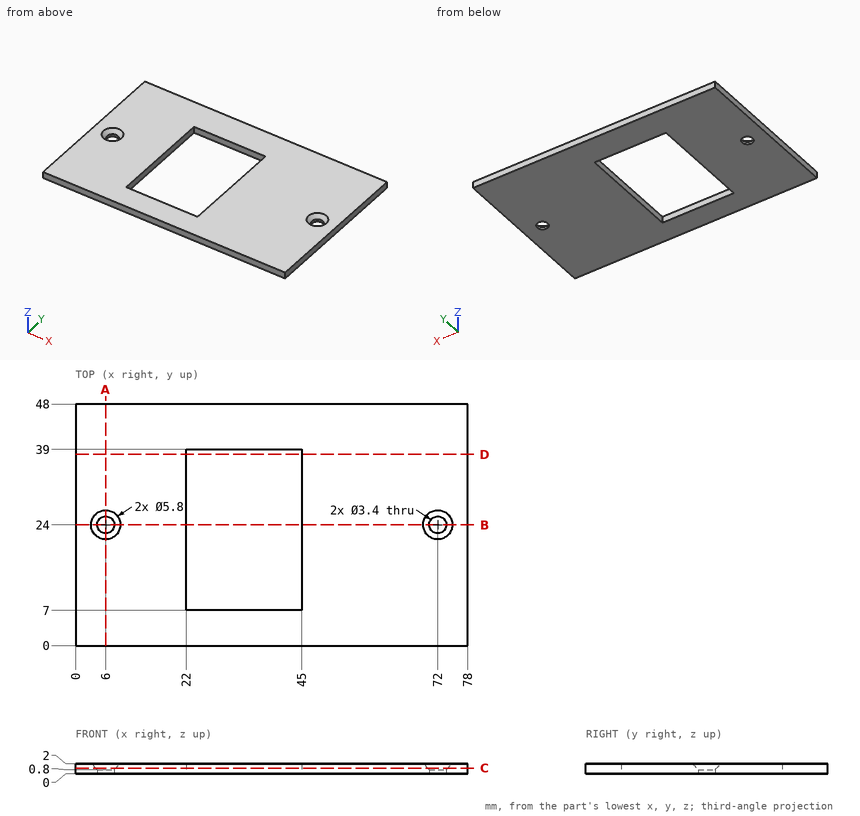
Input: dimensioned drawing with shaded views. Units: mm. Origin: part minimum x, y, z. Give positions to 0.01 mm unless a question says otherwise; leave off trailing zeros. Write each loop counter-clockwise with the first axis right and the second up, starting at its lowest first coordinate (ties: lowest second). Pieces come first, ordered by that corner, then holes. Notation, with made-up numbers: (48.25, 45) -> (68.25, 45) arc R20 cw to (68.25, 68) -> close; hole circle Ø1 at (43, 41). An arc over 180 degrees is marked (long way). Return JSON: item names as keys, results as strings. Group by question number.
1. Section B-B, the plane y = 24. Output: boundary loops of the cut face in (x, z).
2. Section D-D, the plane y = 38. Output: boundary loops of the cut face in (x, z), then the cut area to 3 significant figures.
3. Section C-C, the plane z = 1.1. Output: boundary loops of the cut face in (x, y), then the cut area to 3 significant figures.
4. Pin query (flat end, axial travel): pin 1 Ø10 at (x, y) = (13.5, 23.5) entering from -Z; pin 2 Ø5.5 at (x, y) = (72, 24) entering from +Z. Return the tip coordinate at first contact, or that it passes through.
5. Material intervals for line 1 (X direction, y = 24, z = 0.2); line 2 (Y direction, x = 6, z = 0.55); line 3 (Y direction, x = 37.5, z = 1.4), sorted ascending. Write a range as from..to.
6. Section A-A, the plane x = 6. Output: boundary loops of the cut face in (y, z), then the cut area to 3 significant figures.
Determined:
{
 "1": {"outline": "(0, 0) -> (4.3, 0) -> (4.3, 0.8) -> (3.1, 2) -> (0, 2) -> close; (7.7, 0) -> (22, 0) -> (22, 2) -> (8.9, 2) -> (7.7, 0.8) -> close; (45, 0) -> (70.3, 0) -> (70.3, 0.8) -> (69.1, 2) -> (45, 2) -> close; (73.7, 0) -> (78, 0) -> (78, 2) -> (74.9, 2) -> (73.7, 0.8) -> close"},
 "2": {"outline": "(0, 0) -> (22, 0) -> (22, 2) -> (0, 2) -> close; (45, 0) -> (78, 0) -> (78, 2) -> (45, 2) -> close", "area": "110 mm2"},
 "3": {"outline": "(0, 0) -> (78, 0) -> (78, 48) -> (0, 48) -> close; hole circle Ø4 at (6, 24); hole (22, 7) -> (45, 7) -> (45, 39) -> (22, 39) -> close; hole circle Ø4 at (72, 24)", "area": "2,980 mm2"},
 "4": {"pin 1": "stops at z = 0", "pin 2": "stops at z = 1.85"},
 "5": {"line 1": "x = 0..4.3, 7.7..22, 45..70.3, 73.7..78", "line 2": "y = 0..22.3, 25.7..48", "line 3": "y = 0..7, 39..48"},
 "6": {"outline": "(0, 0) -> (22.3, 0) -> (22.3, 0.8) -> (21.1, 2) -> (0, 2) -> close; (25.7, 0) -> (48, 0) -> (48, 2) -> (26.9, 2) -> (25.7, 0.8) -> close", "area": "87.8 mm2"}
}
